For this review, take the finished solid that the model builds, in its own axes (mm). Face numbers are marked on the shaded views. A direction names the side the tool comes from. Round coordinates to 2 decimals unless told otherwise and drop trailing zeros. Write each loop counter-clockwise with the first axis right and the second up, starting at its lowest first coordinate (ties: lowest second). Pieces come first, ordered by that corner, then holes. Notation, with made-up numbers: (-14.75, 7.5) - (15.25, 7.5) arc R34 ccw to (15.25, 40.5) - close; hole circle Ø2 at (15.25, 47). An arc over 180 degrees is marked (long way). One line per item, written item: value. Start each with the question number.
Q1. Add section C-C on y = 41.5. Write out the cut boundary in (x, z), and give its area (3 significant figures).
Q2. Mouldability with a two-part tool opening along Z and no side actions: class the marked faces 3, 4 and 5 as +Z half, -Z half, draft (parallel to the pull), parting line (faces both ways), or undercut.
Q3. Add section D-D on x = 16.25. Write out the cut boundary in (y, z) (3 decimals), and give its area (3 significant figures).
Q4. Tool access review of the marked faces 1 and 2: name each direction out of +Z, -Z, +X, -X, +Y, -Y from which nothing blocks a thin tool from reaching the whole face with its end or side.
Q5. Add section B-B on x = 5.5. Give the number of separate pieces and of enclosed holes in the cut face, and give its area (3 significant figures).
Q6. For probe 1 along Z at (x, y) = (12.25, 16.5); probe 2 along Y at (x, z) = (17.25, 84.5); probe 3 along Z at (x, y) = (24, 13.5), list the stretches that pass through material, from the lowest coordinate up.
Q7. Add section A-A on y = 9. Write out the cut boundary in (x, z).
Q8. Clearance check with flat-ended pins moving along their axes: pin 1 Ø20 at (y, z) = (84.201, 48.387) entering from -X; pin 2 Ø5.5 at (y, z) = (56.515, 15.875) entering from -X. State where each tip first meets the part, or that it passes through.
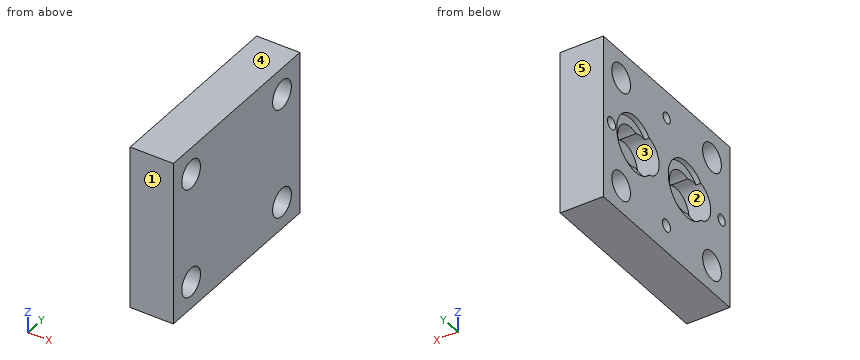
```python
from build123d import *

# Parameters (mm, degrees)
SKETCH1_W           = 112.776
SKETCH1_H           = 96.774
BOSS_EXTRUDE1_DEPTH = 25.4
SKETCH2_R           = 8.334375
CUT_EXTRUDE2_DEPTH  = 151.760715215
SKETCH3_R           = 11.509375
CUT_EXTRUDE3_DEPTH  = 12.7
SKETCH4_R           = 11.509375
CUT_EXTRUDE4_DEPTH  = 12.7
SKETCH5_R           = 16.6497
CUT_EXTRUDE5_DEPTH  = 2.8194
SKETCH6_R           = 3.571875
CUT_EXTRUDE6_DEPTH  = 7.874
SKETCH8_R           = 3.175
CUT_EXTRUDE9_DEPTH  = 7.874


with BuildPart() as part:
    # Sketch1 → Boss-Extrude1 (new body)
    with BuildSketch(Plane.YZ):
        with Locations((56.388, 48.387)):
            Rectangle(SKETCH1_W, SKETCH1_H)
    extrude(amount=BOSS_EXTRUDE1_DEPTH)

    # Sketch2 → Cut-Extrude2 (cut, through all)
    with BuildSketch(Plane.YZ):
        with Locations(Location((15.875, 15.875, 0), (0, 0, 270))):
            Circle(SKETCH2_R)
        with Locations(Location((96.901, 15.875, 0), (0, 0, 270))):
            Circle(SKETCH2_R)
        with Locations(Location((15.875, 80.899, 0), (0, 0, 270))):
            Circle(SKETCH2_R)
        with Locations(Location((96.901, 80.899, 0), (0, 0, 270))):
            Circle(SKETCH2_R)
    extrude(amount=CUT_EXTRUDE2_DEPTH, mode=Mode.SUBTRACT)

    # Sketch3 → Cut-Extrude3 (cut)
    with BuildSketch(Plane.YZ):
        with Locations(Location((28.575, 48.387, 0), (0, 0, 270))):
            Circle(SKETCH3_R)
        with Locations(Location((74.549, 48.387, 0), (0, 0, 270))):
            Circle(SKETCH3_R)
    extrude(amount=CUT_EXTRUDE3_DEPTH, mode=Mode.SUBTRACT)

    # Sketch4 → Cut-Extrude4 (cut)
    with BuildSketch(Plane.YZ):
        with Locations((38.227, 48.387)):
            Circle(SKETCH4_R)
        with Locations((84.201, 48.387)):
            Circle(SKETCH4_R)
    extrude(amount=CUT_EXTRUDE4_DEPTH, mode=Mode.SUBTRACT)

    # Sketch5 → Cut-Extrude5 (cut)
    with BuildSketch(Plane.YZ):
        with Locations((38.227, 48.387)):
            Circle(SKETCH5_R)
        with Locations((84.201, 48.387)):
            Circle(SKETCH5_R)
    extrude(amount=CUT_EXTRUDE5_DEPTH, mode=Mode.SUBTRACT)

    # Sketch6 → Cut-Extrude6 (cut)
    with BuildSketch(Plane.YZ):
        with Locations(Location((105.537, 48.387, 0), (0, 0, 270))):
            Circle(SKETCH6_R)
        with Locations(Location((56.515, 15.875, 0), (0, 0, 270))):
            Circle(SKETCH6_R)
    extrude(amount=CUT_EXTRUDE6_DEPTH, mode=Mode.SUBTRACT)

    # Sketch8 → Cut-Extrude9 (cut)
    with BuildSketch(Plane.YZ):
        with Locations(Location((7.239, 48.387, 0), (0, 0, 270))):
            Circle(SKETCH8_R)
        with Locations(Location((56.261, 80.899, 0), (0, 0, 270))):
            Circle(SKETCH8_R)
    extrude(amount=CUT_EXTRUDE9_DEPTH, mode=Mode.SUBTRACT)


solid = part.part
```
Result set:
1. outline: (0, 0) - (25.4, 0) - (25.4, 96.77) - (0, 96.77) - (0, 64.71) - (2.82, 64.71) - (2.82, 59.42) - (12.7, 59.42) - (12.7, 37.35) - (2.82, 37.35) - (2.82, 32.06) - (0, 32.06) - close
1. area: 2,150 mm^2
2. face 3: undercut
2. face 4: +Z half
2. face 5: draft
3. outline: (0, 0) - (112.776, 0) - (112.776, 96.774) - (0, 96.774) - close; hole circle Ø16.669 at (15.875, 15.875); hole circle Ø16.669 at (15.875, 80.899); hole circle Ø16.669 at (96.901, 15.875); hole circle Ø16.669 at (96.901, 80.899)
3. area: 10,000 mm^2
4. face 1: +Z, -Z, +X, -X, -Y
4. face 2: -X
5. separate pieces: 1
5. enclosed holes: 10
5. area: 8,630 mm^2
6. probe 1: z = 0 to 7.56, 24.19 to 72.59, 89.21 to 96.77
6. probe 2: y = 0 to 8.36, 23.39 to 89.38, 104.42 to 112.78
6. probe 3: z = 0 to 7.89, 23.86 to 72.91, 88.89 to 96.77
7. outline: (0, 0) - (25.4, 0) - (25.4, 11.16) - (0, 11.16) - close; (0, 20.59) - (25.4, 20.59) - (25.4, 76.19) - (0, 76.19) - (0, 51.03) - (7.87, 51.03) - (7.87, 45.75) - (0, 45.75) - close; (0, 85.61) - (25.4, 85.61) - (25.4, 96.77) - (0, 96.77) - close
8. pin 1: stops at x = 12.7
8. pin 2: stops at x = 7.87
